```python
from build123d import *

# Parameters (mm, degrees)
F3_DEPTH  = 20
F4_DEPTH  = 25
F6_DEPTH  = 12.5
F8_W      = 30.1884743385
F8_H      = 13.3378984174
F9_DEPTH  = 25
F11_W     = 24.1160430014
F11_H     = 17.3639170825
F12_DEPTH = 25
F13_R     = 2.25
F14_DEPTH = 25


with BuildPart() as f3:
    # F2 (on line) → F3 (new body)
    with BuildSketch(Plane.YZ.offset(-20)):
        Polygon((-14, 0), (14, 0), (8.5, 4), (-8.5, 4), align=None)
    extrude(amount=F3_DEPTH)

    # F0 (on Top) → F4 (cut)
    with BuildSketch(Plane.XY):
        Polygon((0, -14), (0, -8.5), (-20, -14), align=None)
        Polygon((-20, 14), (0, 8.5), (0, 14), align=None)
    extrude(amount=F4_DEPTH, mode=Mode.SUBTRACT)

    # F5 (on Front) → F6 (cut, symmetric)
    with BuildSketch(Plane.XZ):
        Polygon((-20, 4), (0, 0), (0, 4), align=None)
    extrude(amount=F6_DEPTH, both=True, mode=Mode.SUBTRACT)

    # F8 (on 3pt) → F9 (cut)
    with BuildSketch(Plane(origin=(0.788032027, 2.8655710072, 3.9401601349), x_dir=(0.9871701202, -0.0939145628, -0.1291325238), z_dir=(0.1596720195, 0.5806255255, 0.7983600975))):
        with Locations((-12.3789033387, 7.5781916385)):
            Rectangle(F8_W, F8_H)
    extrude(amount=F9_DEPTH, mode=Mode.SUBTRACT)

    # F11 (on 3pt) → F12 (cut)
    with BuildSketch(Plane(origin=(0.788032027, -2.8655710072, 3.9401601349), x_dir=(0.9871701202, 0.0939145628, -0.1291325238), z_dir=(0.1596720195, -0.5806255255, 0.7983600975))):
        with Locations((-12.0580215007, -6.2219202518)):
            Rectangle(F11_W, F11_H)
    extrude(amount=F12_DEPTH, mode=Mode.SUBTRACT)

    # F13 (on face) → F14 (cut)
    with BuildSketch(Plane(origin=(0, 0, 0), x_dir=(0.9805806757, 0, -0.1961161351), z_dir=(0.1961161351, 0, 0.9805806757))):
        with Locations((-7.55, 0)):
            Circle(F13_R)
    extrude(amount=-F14_DEPTH, mode=Mode.SUBTRACT)


solid = f3.part
```
For this review, take the finished solid that the model builds, in its own axes (mm). Round coordinates to 2 decimals unless told otherwise and drop trailing zeros. Write each loop counter-clockwise with the first axis right and the second up, starting at its lowest first coordinate (ties: lowest second). Pieces come first, ordered by that corner, then holes. Notation, with made-up numbers: (75.5, 56) -> (81.5, 56) arc R31 ccw to (81.5, 84) -> close; hole circle Ø3 at (11.5, 34). An arc over 180 degrees is marked (long way). Use one line per item in the form item = value.
Q1. Consider section B-B (y = -7). State the section outline as (x, z) points, then the cut area to 3 significant figures.
Resolved:
outline = (-20, 0) -> (0, 0) -> (-20, 4) -> close
area = 40.0 mm²
Q2. The part is to be moulded in two halves that separate along X. For faces 1 (the flat face through (-10.14, -0.2, 0)), 2 (the cylindrical face through (-9.758, 0.099, 1.172)), 3 (the flat face through (-20, 0, 2)), 4 (the flat face through (-14.58, 10.16, 1.71)), say which applies: released by +X, released by -X, zero draft, split by the parting line, or undercut.
Resolved:
face_1 = zero draft
face_2 = undercut
face_3 = released by -X
face_4 = released by +X
Q3. Clearance check with flat-ended pins moving along their axes: pin 1 Ø1 at (x, y) = (-12.5, 5.5) entering from -Z; pin 2 Ø2 at (x, z) = (-5.5, 1.5) entering from -Y. State where each tip first meets the part, or that it passes through.
Resolved:
pin_1 = 0
pin_2 = -9.35
Q4. Consider section A-A (z = 2.4). State the section outline as (x, y) points, then the cut area to 3 significant figures.
Resolved:
outline = (-20, -10.7) -> (-12, -8.5) -> (-12, 8.5) -> (-20, 10.7) -> close
area = 154 mm²
Q5. To check wall thickness, follow probe 1 along Y at (x, z) = (-9.75, 0.35); probe 2 along Y at (x, z) = (-7.5, 0.2); probe 3 along Z at (x, y) = (-2, -8.25). State the ranges of each line that lie inside material, in increasing order. Write a range as from..to.
Resolved:
probe_1 = -10.7..-0.86, 0.86..10.7
probe_2 = -10.29..-2.24, 2.24..10.29
probe_3 = 0..0.4
Q6. Consider section C-C (x = -1.75). State the section outline as (y, z) points.
Resolved:
outline = (-8.98, 0) -> (8.98, 0) -> (8.5, 0.35) -> (-8.5, 0.35) -> close
